For this review, take the finished solid that the model builds, in its own axes (mm). A direction names the side the tool comes from. Coordinates: 2 decimals unless noted, no trailing zeros. Write each loop counter-clockwise with the first axis right and the second up, starting at its lowest first coordinate (ties: lowest second). Pieces come first, ordered by that corner, then holes. Notation, with made-up numbers: (33, 19.5) -> (84, 19.5) arc R29 cw to (84, 41.5) -> close; hole circle Ø5 at (36.25, 41). An arc over 180 degrees is marked (long way). Put each result on its own line as item: value. Start each with the question number.
Item 1: Consider section D-D on x = 1.25. Give the boundary of the cut face in (y, z).
Item 2: Consider section A-A on y = 0. Give the boundary of the cut face in (x, z), and give its area (3 significant figures).
Item 3: The part is to be moulded in two halves that separate along X. For faces 4 (the flat face through (-7, 0, 0)), 5 (the flat face through (-10, 0, -10)), 6 (the flat face through (-5, 0, -15)), 7 (the flat face through (0, 0, -10)), say which applies: +X half, -X half, draft (parallel to the pull), parting line (faces both ways), or undercut.
Item 4: Consider section C-C on x = 8. Give the boundary of the cut face in (y, z).
Item 5: To check wall thickness, follow L1, parallel to Z at x = 6.5, y = 3; L2, parallel to Z at x = -2.75, y = -3; L3, parallel to X at y = 0.5, z = 91.5. State the ranges of each line that lie inside material, in increasing order.
Item 6: Consider section B-B on z = 119.5. Give the boundary of the cut face in (x, y), and give its area (3 significant figures).
Item 7: For faces 1 (the cylindrical face through (-1.08, -4.88, 64.09)), 2 (the flat face through (8, 0, -20)), 3 (the flat face through (5, 0, -15)), list the 3-axis set-ups (+Z, -Z, +X, -X, +Y, -Y) from which the entire face can be reached by the end or side of a thin tool; tool diameter is ignored.
Item 8: Insertion check: P1, Ø3, axis at x = 1, y = 1.5, coming from the -Z side; P2, Ø1.5, axis at y = 0, z = 51, coming from the +X side; P3, Ø4, axis at y = -3, z = 19, coming from the +X side. Each pin has a flat end and moves straight along its axis. Give the tip position at first contact, or say it passes through.
```python
from build123d import *

# Parameters (mm, degrees)
SKETCH1_R           = 5
BOSS_EXTRUDE1_DEPTH = 130
SKETCH2_W           = 20
SKETCH2_H           = 10
BOSS_EXTRUDE2_DEPTH = 10
SKETCH3_W           = 5
SKETCH3_H           = 10
BOSS_EXTRUDE3_DEPTH = 10
SKETCH4_W           = 5
SKETCH4_H           = 10
BOSS_EXTRUDE4_DEPTH = 10


with BuildPart() as part:
    # Sketch1 → Boss-Extrude1 (new body)
    with BuildSketch(Plane.XY):
        Circle(SKETCH1_R)
    extrude(amount=BOSS_EXTRUDE1_DEPTH)

    # Sketch2 → Boss-Extrude2 (add)
    with BuildSketch(Plane(origin=(0, 0, 0), x_dir=(-1, 0, 0), z_dir=(0, 0, -1))):
        Rectangle(SKETCH2_W, SKETCH2_H)
    extrude(amount=BOSS_EXTRUDE2_DEPTH)

    # Sketch3 → Boss-Extrude3 (add)
    with BuildSketch(Plane(origin=(0, 0, -10), x_dir=(-1, 0, 0), z_dir=(0, 0, -1))):
        with Locations((-7.5, 0)):
            Rectangle(SKETCH3_W, SKETCH3_H)
    extrude(amount=BOSS_EXTRUDE3_DEPTH)

    # Sketch4 → Boss-Extrude4 (add)
    with BuildSketch(Plane(origin=(0, 0, -10), x_dir=(-1, 0, 0), z_dir=(0, 0, -1))):
        with Locations((7.5, 0)):
            Rectangle(SKETCH4_W, SKETCH4_H)
    extrude(amount=BOSS_EXTRUDE4_DEPTH)


solid = part.part
```
Return value:
1. outline: (-5, -10) -> (5, -10) -> (5, 0) -> (4.84, 0) -> (4.84, 130) -> (-4.84, 130) -> (-4.84, 0) -> (-5, 0) -> close
2. outline: (-10, -20) -> (-5, -20) -> (-5, -10) -> (5, -10) -> (5, -20) -> (10, -20) -> (10, 0) -> (5, 0) -> (5, 130) -> (-5, 130) -> (-5, 0) -> (-10, 0) -> close
2. area: 1,600 mm^2
3. face 4: draft
3. face 5: -X half
3. face 6: undercut
3. face 7: undercut
4. outline: (-5, -20) -> (5, -20) -> (5, 0) -> (-5, 0) -> close
5. L1: -20 to 0
5. L2: -10 to 130
5. L3: -4.97 to 4.97
6. outline: circle Ø10 at (0, 0)
6. area: 78.5 mm^2
7. face 1: +Z
7. face 2: -Z, +X, -X, +Y, -Y
7. face 3: -Z, +Y, -Y
8. P1: z = -10
8. P2: x = 5
8. P3: x = 4.9
